```python
from build123d import *

# Parameters (mm, degrees)
SKETCH1_R             = 2.25
BOSS_EXTRUDE1_DEPTH   = 10
BOSS_EXTRUDE3_DEPTH   = 78
BOSS_EXTRUDE3_2_DEPTH = 78
SKETCH4_R             = 3.5
BOSS_EXTRUDE4_DEPTH   = 10
BOSS_EXTRUDE5_DEPTH   = 8.5
SKETCH5_R             = 3.5
CUT_EXTRUDE1_DEPTH    = 110.542514578
FILLET2_R             = 2
FILLET3_R             = 10


with BuildPart() as part:
    # Sketch1 → Boss-Extrude1 (new body)
    with BuildSketch(Plane.XY):
        with BuildLine():
            Line((15, 19.25), (-15, 19.25))
            Line((-15, 19.25), (-30, 19.25))
            Line((-30, 19.25), (-40, 19.25))
            ThreePointArc((-40, 19.25), (-43.535533906, 17.785533906), (-45, 14.25))
            Line((-45, 14.25), (-45, -14.25))
            ThreePointArc((-45, -14.25), (-43.535533906, -17.785533906), (-40, -19.25))
            Line((-40, -19.25), (-30, -19.25))
            Line((-30, -19.25), (-15, -19.25))
            Line((-15, -19.25), (-8.5, -19.25))
            Line((-8.5, -19.25), (-8.5, -16.75))
            Line((-8.5, -16.75), (-8.5, -11.437329234))
            ThreePointArc((-8.5, -11.437329234), (0, 14.25), (8.5, -11.437329234))
            Line((8.5, -11.437329234), (8.5, -16.75))
            Line((8.5, -16.75), (8.5, -19.25))
            Line((8.5, -19.25), (15, -19.25))
            Line((15, -19.25), (30, -19.25))
            Line((30, -19.25), (40, -19.25))
            ThreePointArc((40, -19.25), (43.535533906, -17.785533906), (45, -14.25))
            Line((45, -14.25), (45, 14.25))
            ThreePointArc((45, 14.25), (43.535533906, 17.785533906), (40, 19.25))
            Line((40, 19.25), (30, 19.25))
            Line((30, 19.25), (15, 19.25))
        make_face()
        with Locations((-15, -15)):
            Circle(SKETCH1_R, mode=Mode.SUBTRACT)
        with Locations((15, -15)):
            Circle(SKETCH1_R, mode=Mode.SUBTRACT)
        with Locations((-15, 15)):
            Circle(SKETCH1_R, mode=Mode.SUBTRACT)
        with Locations((15, 15)):
            Circle(SKETCH1_R, mode=Mode.SUBTRACT)
    extrude(amount=BOSS_EXTRUDE1_DEPTH)

    # Sketch5 → Cut-Extrude1 (cut, through all)
    with BuildSketch(Plane.XY.offset(98)):
        with Locations((-21.5, 0)):
            Circle(SKETCH5_R)
    extrude(amount=-CUT_EXTRUDE1_DEPTH, mode=Mode.SUBTRACT)


with BuildPart() as body_2:
    # Sketch2 → Boss-Extrude3 (new body)
    with BuildSketch(Plane.XY.offset(10)):
        with BuildLine():
            Line((-45, 14.25), (-45, -14.25))
            ThreePointArc((-45, -14.25), (-43.535533906, -17.785533906), (-40, -19.25))
            Line((-40, -19.25), (-28, -19.25))
            Line((-28, -19.25), (-28, 0))
            Line((-28, 0), (-28, 19.25))
            Line((-28, 19.25), (-40, 19.25))
            ThreePointArc((-40, 19.25), (-43.535533906, 17.785533906), (-45, 14.25))
        make_face()
    extrude(amount=BOSS_EXTRUDE3_DEPTH)

    # Sketch4 → Boss-Extrude4 (add)
    with BuildSketch(Plane.XY.offset(88)):
        with BuildLine():
            Line((-45, 14.25), (-45, -14.25))
            ThreePointArc((-45, -14.25), (-43.535533906, -17.785533906), (-40, -19.25))
            Line((-40, -19.25), (-8.5, -19.25))
            Line((-8.5, -19.25), (-8.5, -11.437329234))
            ThreePointArc((-8.5, -11.437329234), (0, 14.25), (8.5, -11.437329234))
            Line((8.5, -11.437329234), (8.5, -19.25))
            Line((8.5, -19.25), (40, -19.25))
            ThreePointArc((40, -19.25), (43.535533906, -17.785533906), (45, -14.25))
            Line((45, -14.25), (45, 14.25))
            ThreePointArc((45, 14.25), (43.535533906, 17.785533906), (40, 19.25))
            Line((40, 19.25), (-40, 19.25))
            ThreePointArc((-40, 19.25), (-43.535533906, 17.785533906), (-45, 14.25))
        make_face()
        with Locations((-21.5, 0)):
            Circle(SKETCH4_R, mode=Mode.SUBTRACT)
    extrude(amount=BOSS_EXTRUDE4_DEPTH)

    # Sketch6 → Boss-Extrude5 (add)
    with BuildSketch(Plane.XY.offset(98)):
        with BuildLine():
            Line((-40, -19.25), (-8.5, -19.25))
            Line((-8.5, -19.25), (-8.5, -11.437329234))
            ThreePointArc((-8.5, -11.437329234), (0, 14.25), (8.5, -11.437329234))
            Line((8.5, -11.437329234), (8.5, -19.25))
            Line((8.5, -19.25), (40, -19.25))
            ThreePointArc((40, -19.25), (43.535533906, -17.785533906), (45, -14.25))
            Line((45, -14.25), (45, 14.25))
            ThreePointArc((45, 14.25), (43.535533906, 17.785533906), (40, 19.25))
            Line((40, 19.25), (-40, 19.25))
            ThreePointArc((-40, 19.25), (-43.535533906, 17.785533906), (-45, 14.25))
            Line((-45, 14.25), (-45, -14.25))
            ThreePointArc((-45, -14.25), (-43.535533906, -17.785533906), (-40, -19.25))
        make_face()
        Polygon((-16.7, 0), (-19.1, 4.156921938), (-23.9, 4.156921938), (-26.3, 0), (-23.9, -4.156921938), (-19.1, -4.156921938), align=None, mode=Mode.SUBTRACT)
    extrude(amount=BOSS_EXTRUDE5_DEPTH)


with BuildPart() as body_3:
    # Sketch2 → Boss-Extrude3 2 (new body)
    with BuildSketch(Plane.XY.offset(10)):
        with BuildLine():
            Line((40, -19.25), (28, -19.25))
            Line((28, -19.25), (28, 0))
            Line((28, 0), (28, 19.25))
            Line((28, 19.25), (40, 19.25))
            ThreePointArc((40, 19.25), (43.535533906, 17.785533906), (45, 14.25))
            Line((45, 14.25), (45, -14.25))
            ThreePointArc((45, -14.25), (43.535533906, -17.785533906), (40, -19.25))
        make_face()
    extrude(amount=BOSS_EXTRUDE3_2_DEPTH)


with BuildPart() as part_1:
    add(part.part)

    # Combine1: union body 2, body 3
    add(body_2.part)
    add(body_3.part)

    # Fillet2
    fillet2_edges = [part_1.edges().sort_by_distance(p)[0] for p in [
        (-28, 0, 88),
    ]]
    fillet(fillet2_edges, radius=FILLET2_R)

    # Fillet3
    # the kernel refuses this fillet: 10 mm, written as the material it adds along each edge
    with BuildSketch(Plane(origin=(28, -19.25, 88), x_dir=(-1, 0, 0), z_dir=(0, 1, 0))) as fillet3_piece_1:
        with BuildLine():
            CenterArc((FILLET3_R, -FILLET3_R), FILLET3_R, 90, 90)
            Line((0, -FILLET3_R), (-FILLET3_R * 0.02, -FILLET3_R))
            Line((-FILLET3_R * 0.02, -FILLET3_R), (-FILLET3_R * 0.02, FILLET3_R * 0.02))
            Line((-FILLET3_R * 0.02, FILLET3_R * 0.02), (FILLET3_R, FILLET3_R * 0.02))
            Line((FILLET3_R, FILLET3_R * 0.02), (FILLET3_R, 0))
        make_face()
    extrude(amount=38.5)
    with BuildSketch(Plane(origin=(-28, -19.25, 10), x_dir=(0, 0, 1), z_dir=(0, 1, 0))) as fillet3_piece_2_section:
        with BuildLine():
            CenterArc((FILLET3_R, FILLET3_R), FILLET3_R, 180, 90)
            Line((0, FILLET3_R), (-FILLET3_R * 0.02, FILLET3_R))
            Line((-FILLET3_R * 0.02, FILLET3_R), (-FILLET3_R * 0.02, -FILLET3_R * 0.02))
            Line((-FILLET3_R * 0.02, -FILLET3_R * 0.02), (FILLET3_R, -FILLET3_R * 0.02))
            Line((FILLET3_R, -FILLET3_R * 0.02), (FILLET3_R, 0))
        make_face()
    fillet3_piece_2 = extrude(amount=38.5, mode=Mode.PRIVATE)
    fillet3_piece_2 = fillet3_piece_2 - Plane(origin=(-21.5, 0, 12.335340949), x_dir=(1, 0, 0), z_dir=(0, 0, 1)) * Cylinder(3.5, 117, mode=Mode.PRIVATE)
    add(fillet3_piece_2)
    with BuildSketch(Plane(origin=(28, 19.25, 10), x_dir=(0, 0, 1), z_dir=(0, -1, 0))) as fillet3_piece_3:
        with BuildLine():
            CenterArc((FILLET3_R, FILLET3_R), FILLET3_R, 180, 90)
            Line((0, FILLET3_R), (-FILLET3_R * 0.02, FILLET3_R))
            Line((-FILLET3_R * 0.02, FILLET3_R), (-FILLET3_R * 0.02, -FILLET3_R * 0.02))
            Line((-FILLET3_R * 0.02, -FILLET3_R * 0.02), (FILLET3_R, -FILLET3_R * 0.02))
            Line((FILLET3_R, -FILLET3_R * 0.02), (FILLET3_R, 0))
        make_face()
    extrude(amount=38.5)


solid = part_1.part
```
Part model, mm, in its own coordinate system. A direction names the side the tool comes from. Coordinates: 2 decimals unless noted, no trailing zeros. Order: outer loops, then holes, each group sorted by start corner. A loop starts at its lowest first (then second) coordinate and runs counter-clockwise, first axis right, second up. Notation, with made-up numbers: (76, 18) - (81, 18) arc R23 ccw to (81, 48) - close; hole circle Ø9 at (3, 74.5). An arc over 180 degrees is marked (long way). Return JSON: item names as keys, results as strings. Group by question number.
Item 1: Pull direction X, two halves, no side cores. Call faces 1 (the face through (31, -19.25, 54)), 2 (the face through (43.57, -17.75, 52.5)), 3 (the face through (-8, 13, 10)): pulls with the +X half, pulls with the -X half, needs draft (parallel to the pull), parting line crosses it, or undercut.
Item 2: Cut at C-C (z = 91). List the corners of the cut face in (x, y), plus the area to 3 significant figures.
Item 3: Cut at B-B (x = 0). List the corners of the cut face in (y, z), plus the area to 4 significant figures.
Item 4: Pin check, flat tips, straight feed: pin 1 (2.5 mm diameter, centred on y = -16.5, z = 94, fed in from +X); pin 2 (8 mm diameter, centred on x = -25.5, y = -14, fed in from -Z); pin 3 (3.5 mm diameter, centred on x = -15, y = 15, fed in from -Z). Stop position of each tip, or through.
Item 5: Cut at A-A (z = 39.5). List the corners of the cut face in (x, y).
Item 6: Which spindle directions (+Z, -Z, +X, -X, +Y, -Y) get a long thin tool onto all of the face, cutting with end or side? Do faces 4 (the face through (8.5, -15, 5)), 5 (the face through (28, 0, 49)), 6 (the face through (16.038, -16.996, 4.93)), 7 (the face through (-22, -4.157, 102)), 8 (the face through (-43.5, 17.82, 52.5)). Say none if no direction does.
Item 7: Cut at D-D (x = -21.5). List the corners of the cut face in (y, z).
Item 8: Drill centre lines: probe 1 along Y at (x, z) = (-15, 8); probe 2 along Z at (x, y) = (16.5, 8.5); probe 3 along X at (y, z) = (0, 7). Where is each one in solid material? Low to high. Write a range as from..to.
Check values:
{
 "1": {"face 1": "needs draft", "face 2": "pulls with the +X half", "face 3": "undercut"},
 "2": {"outline": "(-45, -14.25) arc R5 ccw to (-40, -19.25) - (-8.5, -19.25) - (-8.5, -11.44) arc R14.25 cw (long way) to (8.5, -11.44) - (8.5, -19.25) - (40, -19.25) arc R5 ccw to (45, -14.25) - (45, 14.25) arc R5 ccw to (40, 19.25) - (-40, 19.25) arc R5 ccw to (-45, 14.25) - close; hole circle Ø7 at (-21.5, 0)", "area": "2,670 mm2"},
 "3": {"outline": "(14.25, 0) - (19.25, 0) - (19.25, 10) - (14.25, 10) - close; (14.25, 88) - (19.25, 88) - (19.25, 106.5) - (14.25, 106.5) - close", "area": "142.5 mm2"},
 "4": {"pin 1": "stops at x = 44.9", "pin 2": "stops at z = 0", "pin 3": "stops at z = 88"},
 "5": {"outline": "(-45, -14.25) arc R5 ccw to (-40, -19.25) - (-28, -19.25) - (-28, 19.25) - (-40, 19.25) arc R5 ccw to (-45, 14.25) - close; (28, -19.25) - (40, -19.25) arc R5 ccw to (45, -14.25) - (45, 14.25) arc R5 ccw to (40, 19.25) - (28, 19.25) - close"},
 "6": {"face 4": "+Z, -Z, -Y", "face 5": "+Y, -Y", "face 6": "-Z", "face 7": "+Z", "face 8": "+Z, -Z, -X, +Y"},
 "7": {"outline": "(-19.25, 0) - (-3.5, 0) - (-3.5, 10.63) - (-19.25, 10.63) - close; (-19.25, 88) - (-3.5, 88) - (-3.5, 98) - (-4.16, 98) - (-4.16, 106.5) - (-19.25, 106.5) - close; (3.5, 0) - (19.25, 0) - (19.25, 10.63) - (3.5, 10.63) - close; (3.5, 88) - (19.25, 88) - (19.25, 106.5) - (4.16, 106.5) - (4.16, 98) - (3.5, 98) - close"},
 "8": {"probe 1": "y = -19.25..-17.25, -12.75..12.75, 17.25..19.25", "probe 2": "z = 0..10, 88..106.5", "probe 3": "x = -45..-25, -18..-14.25, 14.25..45"}
}
